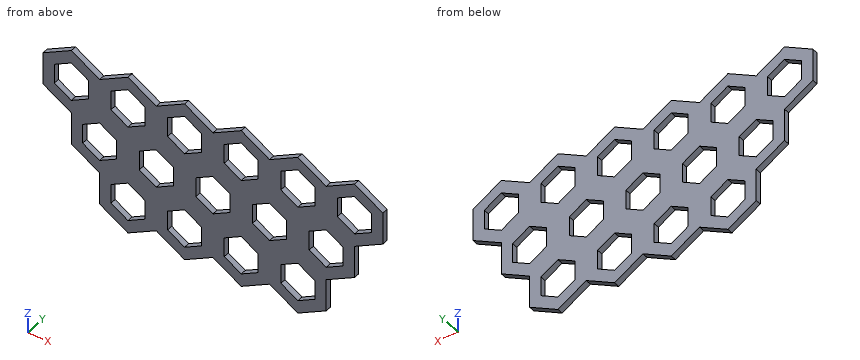
from build123d import *

# Parameters (mm, degrees)
BOSS_EXTRUDE2_DEPTH = 0.5


with BuildPart() as part:
    # Sketch1 → Boss-Extrude2 (new body)
    with BuildSketch(Plane(origin=(0, 0, 0), x_dir=(1, 0, 0), z_dir=(0, 1, 0))):
        Polygon((-2.5, -7.216878365), (0, -5.773502692), (0, -2.886751346), (-2.5, -1.443375673), (-5, -2.886751346), (-5, -5.773502692), align=None)
        Polygon((-1, -3.464101615), (-2.5, -2.598076211), (-4, -3.464101615), (-4, -5.196152423), (-2.5, -6.062177826), (-1, -5.196152423), align=None, mode=Mode.SUBTRACT)
        Polygon((-5, -11.547005384), (-2.5, -10.103629711), (-2.5, -7.216878365), (-5, -5.773502692), (-7.5, -7.216878365), (-7.5, -10.103629711), align=None)
        Polygon((-3.5, -7.794228634), (-5, -6.92820323), (-6.5, -7.794228634), (-6.5, -9.526279442), (-5, -10.392304845), (-3.5, -9.526279442), align=None, mode=Mode.SUBTRACT)
        Polygon((0, -11.547005384), (2.5, -10.103629711), (2.5, -7.216878365), (0, -5.773502692), (-2.5, -7.216878365), (-2.5, -10.103629711), align=None)
        Polygon((1.5, -7.794228634), (0, -6.92820323), (-1.5, -7.794228634), (-1.5, -9.526279442), (0, -10.392304845), (1.5, -9.526279442), align=None, mode=Mode.SUBTRACT)
        Polygon((5, -11.547005384), (7.5, -10.103629711), (7.5, -7.216878365), (5, -5.773502692), (2.5, -7.216878365), (2.5, -10.103629711), align=None)
        Polygon((6.5, -7.794228634), (5, -6.92820323), (3.5, -7.794228634), (3.5, -9.526279442), (5, -10.392304845), (6.5, -9.526279442), align=None, mode=Mode.SUBTRACT)
        Polygon((2.5, -7.216878365), (5, -5.773502692), (5, -2.886751346), (2.5, -1.443375673), (0, -2.886751346), (0, -5.773502692), align=None)
        Polygon((4, -3.464101615), (2.5, -2.598076211), (1, -3.464101615), (1, -5.196152423), (2.5, -6.062177826), (4, -5.196152423), align=None, mode=Mode.SUBTRACT)
        Polygon((2.5, -1.443375673), (2.5, 1.443375673), (0, 2.886751346), (-2.5, 1.443375673), (-2.5, -1.443375673), (0, -2.886751346), align=None)
        Polygon((1.5, 0.866025404), (0, 1.732050808), (-1.5, 0.866025404), (-1.5, -0.866025404), (0, -1.732050808), (1.5, -0.866025404), align=None, mode=Mode.SUBTRACT)
        Polygon((7.5, -1.443375673), (7.5, 1.443375673), (5, 2.886751346), (2.5, 1.443375673), (2.5, -1.443375673), (5, -2.886751346), align=None)
        Polygon((6.5, 0.866025404), (5, 1.732050808), (3.5, 0.866025404), (3.5, -0.866025404), (5, -1.732050808), (6.5, -0.866025404), align=None, mode=Mode.SUBTRACT)
        Polygon((7.5, -7.216878365), (10, -5.773502692), (10, -2.886751346), (7.5, -1.443375673), (5, -2.886751346), (5, -5.773502692), align=None)
        Polygon((9, -3.464101615), (7.5, -2.598076211), (6, -3.464101615), (6, -5.196152423), (7.5, -6.062177826), (9, -5.196152423), align=None, mode=Mode.SUBTRACT)
        Polygon((10, -11.547005384), (12.5, -10.103629711), (12.5, -7.216878365), (10, -5.773502692), (7.5, -7.216878365), (7.5, -10.103629711), align=None)
        Polygon((11.5, -7.794228634), (10, -6.92820323), (8.5, -7.794228634), (8.5, -9.526279442), (10, -10.392304845), (11.5, -9.526279442), align=None, mode=Mode.SUBTRACT)
        Polygon((22.5, -10.103629711), (22.5, -7.216878365), (20, -5.773502692), (17.5, -7.216878365), (17.5, -10.103629711), (20, -11.547005384), align=None)
        Polygon((21.5, -7.794228634), (20, -6.92820323), (18.5, -7.794228634), (18.5, -9.526279442), (20, -10.392304845), (21.5, -9.526279442), align=None, mode=Mode.SUBTRACT)
        Polygon((15, -11.547005384), (17.5, -10.103629711), (17.5, -7.216878365), (15, -5.773502692), (12.5, -7.216878365), (12.5, -10.103629711), align=None)
        Polygon((16.5, -7.794228634), (15, -6.92820323), (13.5, -7.794228634), (13.5, -9.526279442), (15, -10.392304845), (16.5, -9.526279442), align=None, mode=Mode.SUBTRACT)
        Polygon((20, -5.773502692), (20, -2.886751346), (17.5, -1.443375673), (15, -2.886751346), (15, -5.773502692), (17.5, -7.216878365), align=None)
        Polygon((19, -3.464101615), (17.5, -2.598076211), (16, -3.464101615), (16, -5.196152423), (17.5, -6.062177826), (19, -5.196152423), align=None, mode=Mode.SUBTRACT)
        Polygon((12.5, -7.216878365), (15, -5.773502692), (15, -2.886751346), (12.5, -1.443375673), (10, -2.886751346), (10, -5.773502692), align=None)
        Polygon((14, -3.464101615), (12.5, -2.598076211), (11, -3.464101615), (11, -5.196152423), (12.5, -6.062177826), (14, -5.196152423), align=None, mode=Mode.SUBTRACT)
        Polygon((17.5, -1.443375673), (17.5, 1.443375673), (15, 2.886751346), (12.5, 1.443375673), (12.5, -1.443375673), (15, -2.886751346), align=None)
        Polygon((16.5, 0.866025404), (15, 1.732050808), (13.5, 0.866025404), (13.5, -0.866025404), (15, -1.732050808), (16.5, -0.866025404), align=None, mode=Mode.SUBTRACT)
        Polygon((12.5, -1.443375673), (12.5, 1.443375673), (10, 2.886751346), (7.5, 1.443375673), (7.5, -1.443375673), (10, -2.886751346), align=None)
        Polygon((11.5, 0.866025404), (10, 1.732050808), (8.5, 0.866025404), (8.5, -0.866025404), (10, -1.732050808), (11.5, -0.866025404), align=None, mode=Mode.SUBTRACT)
    extrude(amount=BOSS_EXTRUDE2_DEPTH)


solid = part.part
Can you work these out from the model? Positions are in its coordinate system, mm. Give positions to 0.01 mm unless a question says otherwise; leave off trailing zeros. Order: outer loops, then holes, each group sorted by start corner. A loop starts at its lowest first (then second) coordinate and runs counter-clockwise, first axis right, second up. Notation, with made-up numbers: M -35.5,41 L -10.5,41 A24 ccw -10.5,68 Z; hole C 3.5,38.5 d2. An arc over 180 degrees is marked long. Use a Markdown table: item, result. Add a question column.
Item 1: Suppose I cut it at A-A (x = 3). List the corners of the cut face in (y, z) for me.
Item 2: If I drill on L1, parallel to X at y = 0.1, z = -0.75; L2, parallel to Z at x = 9.75, y = 0.45; L3, parallel to Z at x = 0.5, y = 0.05, over which ranges is the centre line in solid material (lowest first)? Write a range as [from, to].
Item 3: Suppose I cut it at C-C (z = 9.25). List the corners of the cut face in (x, y) for me, then the cut area to 3 significant figures.
Item 4: Suppose I cut it at D-D (y = 0.25). Count the separate pieces of the cut face and the enclosed holes in it, then the cut area to 3 significant figures.
Item 5: Suppose I cut it at B-B (z = 4.75). List the corners of the cut face in (x, y) for me.
Answer sheet:
| question | item | result |
|---|---|---|
| 1 | outline | M 0,-1.73 L 0.5,-1.73 L 0.5,2.89 L 0,2.89 Z; M 0,5.77 L 0.5,5.77 L 0.5,10.39 L 0,10.39 Z |
| 2 | L1 | x = [-2.5, -1.5], [1.5, 3.5], [6.5, 8.5], [11.5, 13.5], [16.5, 17.5] |
| 2 | L2 | z = [-2.74, -1.59], [1.59, 7.07], [10.25, 11.4] |
| 2 | L3 | z = [-2.6, -1.44], [1.44, 7.22], [10.1, 11.26] |
| 3 | outline | M -7.5,0 L -6.5,0 L -6.5,0.5 L -7.5,0.5 Z; M -3.5,0 L -1.5,0 L -1.5,0.5 L -3.5,0.5 Z; M 1.5,0 L 3.5,0 L 3.5,0.5 L 1.5,0.5 Z; M 6.5,0 L 8.5,0 L 8.5,0.5 L 6.5,0.5 Z; M 11.5,0 L 13.5,0 L 13.5,0.5 L 11.5,0.5 Z; M 16.5,0 L 18.5,0 L 18.5,0.5 L 16.5,0.5 Z; M 21.5,0 L 22.5,0 L 22.5,0.5 L 21.5,0.5 Z |
| 3 | area | 6.00 mm² |
| 4 | separate pieces | 1 |
| 4 | enclosed holes | 15 |
| 4 | area | 208 mm² |
| 5 | outline | M -5,0 L -4,0 L -4,0.5 L -5,0.5 Z; M -1,0 L 1,0 L 1,0.5 L -1,0.5 Z; M 4,0 L 6,0 L 6,0.5 L 4,0.5 Z; M 9,0 L 11,0 L 11,0.5 L 9,0.5 Z; M 14,0 L 16,0 L 16,0.5 L 14,0.5 Z; M 19,0 L 20,0 L 20,0.5 L 19,0.5 Z |
